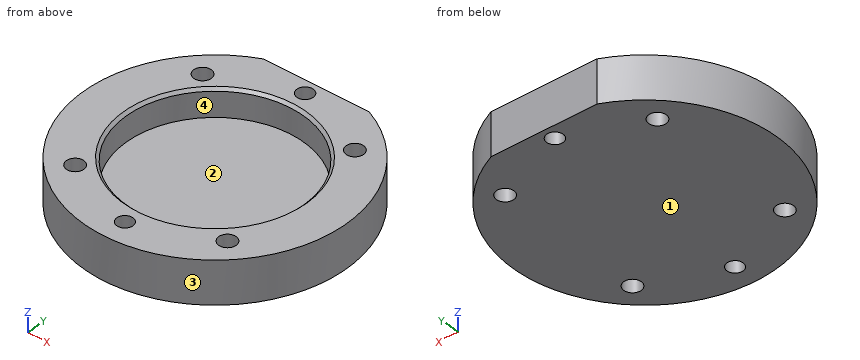
from build123d import *

# Parameters (mm, degrees)
BASE_EXTRUDE_DEPTH = 8.001
HOLE1_D            = 3.048
HOLE2_D            = 3.2512
CIRPATTERN1_COUNT  = 4
HOLE3_D            = 2.99974
SKETCH8_R          = 16.51
CUT_EXTRUDE1_DEPTH = 5.1562
CHAMFER1_SIZE      = 0.508


with BuildPart() as part:
    # Sketch1 → Base-Extrude (new body)
    with BuildSketch(Plane.XY):
        with BuildLine():
            Line((-9.8298, 22.4536), (9.8298, 22.4536))
            ThreePointArc((9.8298, 22.4536), (0, -24.511), (-9.8298, 22.4536))
        make_face()
    extrude(amount=BASE_EXTRUDE_DEPTH)

    # Hole1 (through all)
    with Locations(Plane.XY.offset(8.001)):
        with Locations((0, 19.99996)):
            Hole(HOLE1_D / 2)

    # Hole2 (through all)
    with Locations(Plane.XY.offset(8.001)):
        with Locations((-14.142107339, 14.142107339)):
            hole2 = Hole(HOLE2_D / 2)

    # CirPattern1: Hole2 ×4 about axis
    cirpattern1_axis = Axis((0, 0, 0), (0, 0, 1))
    for i in range(1, CIRPATTERN1_COUNT):
        add(hole2.rotate(cirpattern1_axis, i * 360 / CIRPATTERN1_COUNT), mode=Mode.SUBTRACT)

    # Hole3 (through all)
    with Locations(Plane.XY.offset(8.001)):
        with Locations((0, -20.0025)):
            Hole(HOLE3_D / 2)

    # Sketch8 → Cut-Extrude1 (cut)
    with BuildSketch(Plane.XY.offset(8.001)):
        Circle(SKETCH8_R)
    extrude(amount=-CUT_EXTRUDE1_DEPTH, mode=Mode.SUBTRACT)

    # Chamfer1
    chamfer1_edges = [part.edges().sort_by_distance(p)[0] for p in [
        (-16.51, 0, 8.001),
    ]]
    chamfer(chamfer1_edges, length=CHAMFER1_SIZE)


solid = part.part
Verification items for the finished model (mm, model axes). Face numbers are marked on the shaded views. Round coordinates to 2 decimals unless told otherwise and drop trailing zeros. Loops run counter-clockwise (first coordinate to the right, second up) from the corner with the lowest first, then second, coordinate; pieces in that order, holes last. Notation, with made-up numbers: M 43.5,-22 L 53.5,-22 A21 cw 53.5,13 Z; hole C 12,44.5 d3. An arc over 180 degrees is marked long. Write each question's results on one line, items separated by ' | '.
1) Mould release check, pull along X, two halves, no side actions. Record for the marked faces 1, 2, 3 and 4: released by +X, released by -X, zero draft, split by the parting line, or undercut.
Checks:
face 1: zero draft | face 2: undercut | face 3: split by the parting line | face 4: undercut
2) Gauge pin test, flat ends, axial feed: P1, Ø2.5, axis at x = -14.14, y = -14.14, coming from the -Z side; P2, Ø20, axis at x = 0, y = 0, coming from the +Z side; P3, Ø3, axis at x = 19.5, z = 6, coming from the -Y side; P4, Ø2, axis at y = -5.5, z = 1.5, coming from the +X side. Record the tip position at first contact, or that the pin passes through.
Checks:
P1: passes through | P2: stops at z = 2.84 | P3: stops at y = -16.64 | P4: stops at x = 24.09
3) Section check C-C on z = 3.5. Record the boundary of the cut face in (x, y), then the cut area to 3 significant figures.
Checks:
outline: M -9.83,22.45 A24.51 ccw long 9.83,22.45 Z; hole C 0,0 d33.02; hole C -14.14,-14.14 d3.25; hole C -14.14,14.14 d3.25; hole C 0,20 d3.05; hole C 0,-20 d3; hole C 14.14,-14.14 d3.25; hole C 14.14,14.14 d3.25 | area: 956 mm2
4) Section check B-B on y = 0. Record the boundary of the cut face in (x, z), then the cut area to 3 significant figures.
Checks:
outline: M -24.51,0 L 24.51,0 L 24.51,8 L 17.02,8 L 16.51,7.49 L 16.51,2.84 L -16.51,2.84 L -16.51,7.49 L -17.02,8 L -24.51,8 Z | area: 222 mm2
5) Scan lines: L1, parallel to Z at x = 10, y = -4; L2, parallel to X at y = -15, z = 4.25; L3, parallel to Y at x = 7, z = 7. Record each from-to range of solid material in increasing order. Write a range as from..to.
Checks:
L1: z = 0..2.84 | L2: x = -19.39..-15.52, -12.76..-6.9, 6.9..12.76, 15.52..19.39 | L3: y = -23.49..-14.95, 14.95..22.45
6) Section check A-A on x = 0. Record the boundary of the cut face in (y, z), then the cut area to 3 significant figures.
Checks:
outline: M -24.51,0 L -21.5,0 L -21.5,8 L -24.51,8 Z; M -18.5,0 L 18.48,0 L 18.48,8 L 17.02,8 L 16.51,7.49 L 16.51,2.84 L -16.51,2.84 L -16.51,7.49 L -17.02,8 L -18.5,8 Z; M 21.52,0 L 22.45,0 L 22.45,8 L 21.52,8 Z | area: 157 mm2
